Job drawing, mm, ordinate dimensions from the low corner. One solid piece. Give positions to 0.01 mm unless a question says otherwise; leave off trailing zeros. Loops run counter-clockwise (first coordinate to the right, second up) from the corner with the lowest first, then second, coordinate; pieces in that order, holes last. Notation, with made-up numbers: M -31.5,-28.5 L -1.5,-28.5 A32 cw -1.5,3.5 Z; hole C 80.25,69 d10. An arc over 180 degrees is marked long. Answer in a Markdown table with one row per item.
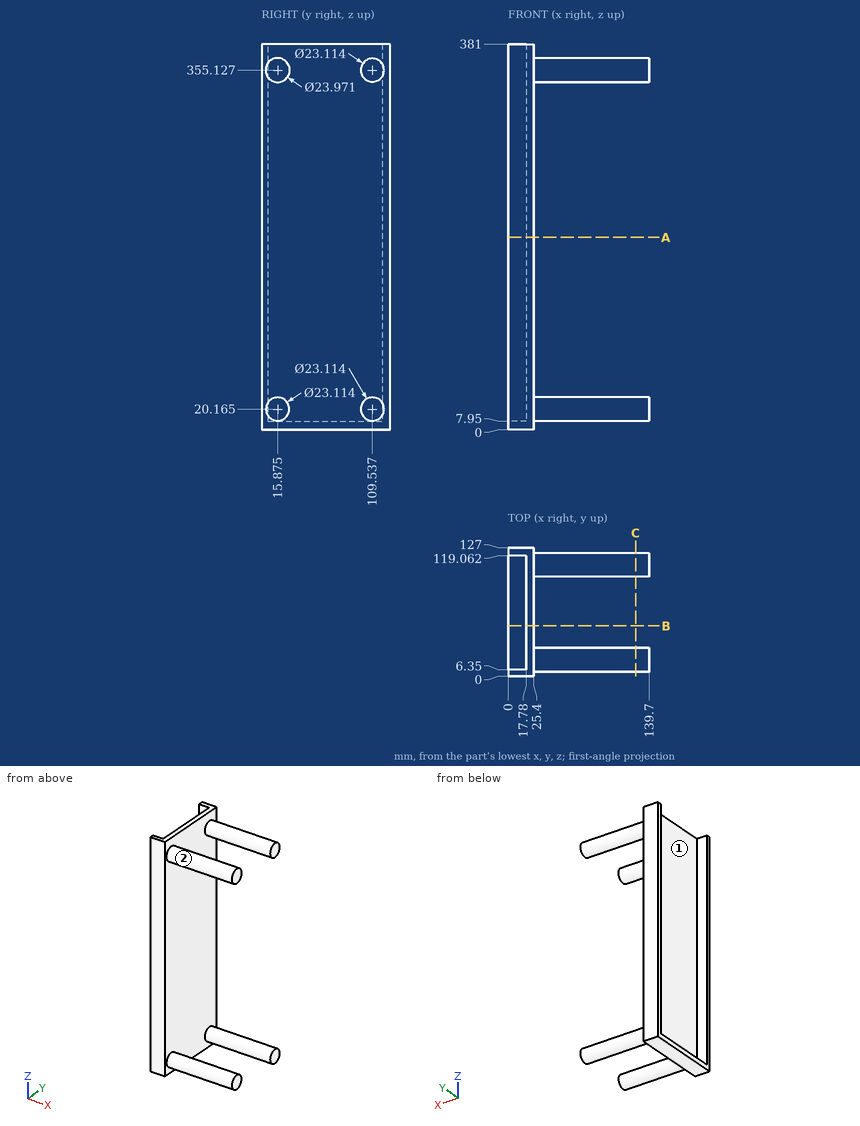
(1) Saw through at A-A (z = 190). Write the cut outline in (x, y).
Recorded:
| item | result |
|---|---|
| outline | M 0,0 L 25.4,0 L 25.4,127 L 0,127 L 0,119.06 L 17.78,119.06 L 17.78,6.35 L 0,6.35 Z |
(2) Drill centre lines: line 1 along X through (y, z) = (36.5, 70); line 2 along Z through (x, y) = (14, 78.5); line 3 along X through (y, z) = (120, 153). Where is each one in solid material? Low to high.
Recorded:
| item | result |
|---|---|
| line 1 | x = 17.78 to 25.4 |
| line 2 | z = 0 to 7.95 |
| line 3 | x = 0 to 25.4 |
(3) Saw through at C-C (x = 126). Write the cut outline in (y, z) (1 decimal).
Recorded:
| item | result |
|---|---|
| outline | C 15.9,355.1 d24; C 15.9,20.2 d23.1; C 109.5,20.2 d23.1; C 109.5,355.1 d23.1 |
(4) Saw through at B-B (y = 49.5). Write the cut outline in (x, z).
Recorded:
| item | result |
|---|---|
| outline | M 0,0 L 25.4,0 L 25.4,381 L 17.78,381 L 17.78,7.95 L 0,7.95 Z |
(5) Pull direction Y, two halves, no side cores. Call the marked faces 1 and 2: +Y half, -Y half, draft (parallel to the pull), parting line (faces both ways), or undercut.
Recorded:
| item | result |
|---|---|
| face 1 | undercut |
| face 2 | undercut |
(6) Pin check, flat tips, straight feed: pin 1 Ø10 at (y, z) = (61.5, 118.5) entering from +X; pin 2 Ø1 at (x, y) = (58, 111.5) entering from +Z; pin 3 Ø8 at (x, y) = (81, 112.5) entering from -Z. Stop position of each tip, or through.
Recorded:
| item | result |
|---|---|
| pin 1 | stops at x = 25.4 |
| pin 2 | stops at z = 366.59 |
| pin 3 | stops at z = 8.61 |
